The model under review builds one solid part; all positions refer to its coordinate system, in mm. Face numbers are marked on the shaded views. Round coordinates to 2 decimals unless told otherwise and drop trailing zeros. Write each loop counter-clockwise with the first axis right and the second up, starting at its lowest first coordinate (ties: lowest second). Pieces come first, ordered by that corner, then holes. Notation, with made-up numbers: M 15,43.5 L 26,43.5 A34 cw 26,81.5 Z; hole C 55,41.25 d9. An arc over 180 degrees is marked long. Write item = value, one per line. Start each with the question number.
Item 1: Take a section at D-D, the plane x = 9. Give the boundary of the cut face in (y, z), plus the area to 3 significant figures.
Item 2: Take a section at C-C, the plane z = 215. Give the boundary of the cut face in (x, y).
Item 3: The part is to be moulded in two halves that separate along Y. For the marked faces 1, 2, 3 and 4, say which applies: +Y half, -Y half, draft (parallel to the pull), parting line (faces both ways), or undercut.
Item 4: Take a section at B-B, the plane y = 18. Give the boundary of the cut face in (x, z).
Item 5: Take a section at A-A, the plane x = 64.5. Give the boundary of the cut face in (y, z), plus the area to 3 significant figures.
Item 6: To check wall thickness, follow line 1 along Z through (x, y) = (52, 42.5); line 2 along X through (y, z) = (42.5, 199); line 3 along Z through (x, y) = (31, 17). State the ranges of each line that lie inside material, in increasing order.
Item 7: For pin 1 Ø12 at (x, y) = (8, 49) entering from +Z; pin 2 Ø2 at (x, z) = (14.5, 123) entering from -Y; pin 3 Ø5.5 at (x, z) = (33, 226.5) entering from +Y; pin 4 Ø7.5 at (x, z) = (42.5, 225.5) entering from -Y, all flat-tipped, find the tip position at first contact; note any pin that passes through.
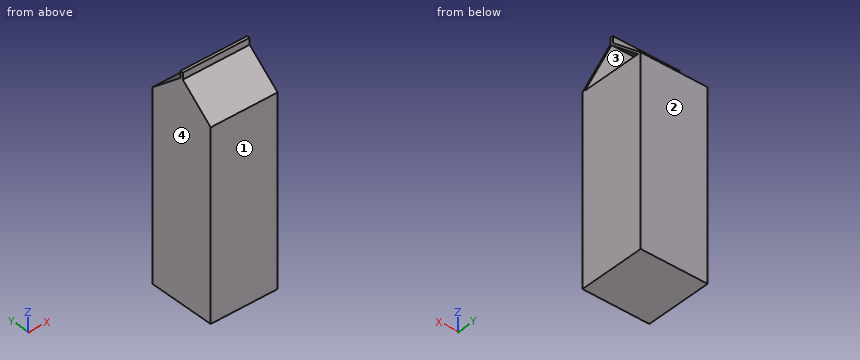
from build123d import *

# Parameters (mm, degrees)
F1_DEPTH = 70


with BuildPart() as f1:
    # F0 (on Right) → F1 (new body)
    with BuildSketch(Plane.YZ):
        Polygon((0, 194), (0, 0), (70, 0), (70, 194), (36.5, 222.109838), (36.5, 229), (33.5, 229), (33.5, 222.109838), align=None)
    extrude(amount=F1_DEPTH)

    # F2 (on face) → F5 section 0
    with BuildSketch(Plane.YZ.offset(70), mode=Mode.PRIVATE) as f5_s0:
        Polygon((35, 220.757673), (3.111448, 194), (66.888552, 194), align=None)
    loft([f5_s0.sketch, Vertex(35, 35, 220.757673)], mode=Mode.SUBTRACT)


solid = f1.part
Response values:
q1.outline = M 0,0 L 70,0 L 70,194 L 36.5,222.11 L 36.5,229 L 33.5,229 L 33.5,222.11 L 0,194 Z
q1.area = 14,600 mm2
q2.outline = M 0,25.03 L 70,25.03 L 70,28.14 L 42.53,28.14 L 42.53,41.86 L 70,41.86 L 70,44.97 L 0,44.97 Z
q3.face_1 = -Y half
q3.face_2 = +Y half
q3.face_3 = undercut
q3.face_4 = draft
q4.outline = M 0,0 L 70,0 L 70,194 L 53.66,206.49 L 70,206.49 L 70,209.1 L 0,209.1 Z
q5.outline = M 0,0 L 70,0 L 70,194 L 36.5,222.11 L 36.5,229 L 33.5,229 L 33.5,222.11 L 0,194 Z; hole M 8.12,198.2 L 61.88,198.2 L 35,220.76 Z
q5.area = 14,000 mm2
q6.line_1 = 0 to 207.76, 214.46 to 217.08
q6.line_2 = 0 to 63.46
q6.line_3 = 0 to 208.26
q7.pin_1 = 216.66
q7.pin_2 = 0
q7.pin_3 = 36.5
q7.pin_4 = 33.07
